Geometry check sheet. Reference: the model listing, model coordinates, mm. Round coordinates to 2 decimals unless told otherwise and drop trailing zeros. Order: outer loops, then holes, each group sorted by start corner. A loop starts at its lowest first (then second) coordinate and runs counter-clockwise, first axis right, second up. Notation, with made-up numbers: (11.25, -8.75) - (49.25, -8.75) arc R18 ccw to (49.25, -2.75) - close; hole circle Ø5 at (7, -15.5). An arc over 180 degrees is marked (long way). Return JSON: item names as keys, results as strings. Group by question number.
Q1. Material ranges on line 1 along Z through (x, y) = (0, -3.5); line 2 along Z through (x, y) = (-32, 6), recorded low to high.
Q2. Gauge pin test, flat ends, axial feed: pin 1 Ø5 at (x, y) = (-6.5, 3) entering from +Z; pin 2 Ø2.5 at (x, z) = (0, 45.5) entering from -Y; pin 3 Ø3 at (x, y) = (15, -0.5) entering from +Z; pin 4 Ø6 at (y, z) = (2.5, 9) entering from +X (3 decimals). Record the tip position at first contact, or that the pin passes through.
Q3. Sectioned sample at A-A, the plane z = 0. Record the cut outline in (x, y).
Q4. Sectioned sample at C-C, the plane y = -2.5. Give the number of separate pieces and of enclosed holes in the cut face, then the cut area to 3 significant figures.
Q5. Sectioned sample at B-B, the plane x = -12. Record the cut outline in (y, z), then the cut area to 3 significant figures.
Q6. Sectioned sample at D-D, the plane z = -45.5. Record the cut outline in (x, y).
Q7. Draft check along X on faces 1 (the flat face through (-26, 7, -33)), 2 (the cylindrical face through (-6.44, 0.1, -49.08)), 3 (the cylindrical face through (43.27, -0.1, -0.29)). Enter one of: pulls with the +X half, pulls with the -X half, needs draft (parallel to the pull), parting line crosses it, or undercut.
Autodesk Inventor part; units mm, degrees
ref_plane "YZ Plane" through (0, 0, 0) normal (1, 0, 0) x (0, 1, 0)
ref_plane "XZ Plane" through (0, 0, 0) normal (0, 1, 0) x (-1, 0, 0)
ref_plane "XY Plane" through (0, 0, 0) normal (0, 0, 1) x (1, 0, 0)
sketch "Sketch1" plane through (0, 0, 0) normal (0, 0, 1) x (1, 0, 0)
  line L0 (0, 9.8) -> (0, -9.8) construction
  line L1 (-9.9, 0) -> (59.4, 0) construction
  line L2 (41.5, 7) -> (41.5, -7)
  line L3 (41.5, -7) -> (49.5, -7)
  line L4 (49.5, -7) -> (49.5, 7)
  line L5 (49.5, 7) -> (41.5, 7)
  line L6 (45.5, 7) -> (45.5, -7) construction
  point P0 (0, 0)
  dimension "d0" = 45.5
  dimension "d1" = 4
  dimension "d2" = 14
revolve "Revolution1" add sketch "Sketch1" angle 360 about axis through (0, 0, 0) along (0, -1, 0)
sketch "Sketch2" plane through (0, 7, 0) normal (0, 1, 0) x (1, 0, 0)
  line L0 (0, 69.3) -> (0, -69.3) construction
  line L1 (69.3, 0) -> (-69.3, 0) construction
  circle A0 centre (0, 0) radius 45.5 construction
  circle A1 centre (0, 0) radius 49.5 construction
  circle A2 centre (0, 0) radius 41.5 construction
  point P0 (-45.5, 0)
  point P1 (-32.1734, -32.1734)
  point P2 (0, -45.5)
  point P3 (32.1734, -32.1734)
  point P4 (45.5, 0)
  point P5 (32.1734, 32.1734)
  point P6 (0, 45.5)
  point P7 (-32.1734, 32.1734)
  dimension "d4" = 4
  dimension "d5" = 4
  dimension "d8" = 360
hole "Hole1" at (-45.5, 7, 0) at (-32.1734, 7, 32.1734) at (0, 7, 45.5) at (32.1734, 7, 32.1734) at (45.5, 7, 0) at (32.1734, 7, -32.1734) at (0, 7, -45.5) at (-32.1734, 7, -32.1734) direction (0, -1, 0) diameter 4.5 end through all
equation "\"d4\" = d5"
properties part number "Adapter_bearing_joint"
Reply:
{
 "1": {"line 1": "-49.5 to -47.75, -43.25 to -41.5, 41.5 to 43.25, 47.75 to 49.5", "line 2": "-37.77 to -34.42, -29.93 to -26.42, 26.42 to 29.93, 34.42 to 37.77"},
 "2": {"pin 1": "z = 49.34", "pin 2": "through", "pin 3": "z = 47.62", "pin 4": "x = 49.135"},
 "3": {"outline": "(-49.5, -7) - (-47.75, -7) - (-47.75, 7) - (-49.5, 7) - close; (-43.25, -7) - (-41.5, -7) - (-41.5, 7) - (-43.25, 7) - close; (41.5, -7) - (43.25, -7) - (43.25, 7) - (41.5, 7) - close; (47.75, -7) - (49.5, -7) - (49.5, 7) - (47.75, 7) - close"},
 "4": {"separate pieces": "1", "enclosed holes": "9", "area": "2,160 mm^2"},
 "5": {"outline": "(-7, -48.02) - (7, -48.02) - (7, -39.73) - (-7, -39.73) - close; (-7, 39.73) - (7, 39.73) - (7, 48.02) - (-7, 48.02) - close", "area": "232 mm^2"},
 "6": {"outline": "(-19.49, -7) - (-2.25, -7) - (-2.25, 7) - (-19.49, 7) - close; (2.25, -7) - (19.49, -7) - (19.49, 7) - (2.25, 7) - close"},
 "7": {"face 1": "needs draft", "face 2": "parting line crosses it", "face 3": "undercut"}
}
